from build123d import *

# Parameters (mm, degrees)
SKETCH2_W           = 18
SKETCH2_H           = 18
BOSS_EXTRUDE1_DEPTH = 8
BOSS_EXTRUDE1_TAPER = 11
FILLET1_R           = 1
SHELL1_OUTLINE_W    = 13.241242282
SHELL1_OUTLINE_H    = 13.241242282
SHELL1_DEPTH        = 7
SHELL1_DRAFT        = 11
SKETCH3_R           = 2.8
BOSS_EXTRUDE2_DEPTH = 5.5
SKETCH4_W           = 1.161559242
SKETCH4_H           = 1.419220379
SKETCH4_H_2         = 1.161559242
SKETCH4_W_2         = 1.419220379
CUT_EXTRUDE1_DEPTH  = 5.5


# Read off the part's stored shape, not the designer's step: Shell1
with BuildPart() as part:
    # Sketch2 → Boss-Extrude1 (new body)
    with BuildSketch(Plane(origin=(0, 0, 0), x_dir=(1, 0, 0), z_dir=(0, 1, 0))):
        Rectangle(SKETCH2_W, SKETCH2_H)
    extrude(amount=BOSS_EXTRUDE1_DEPTH, taper=BOSS_EXTRUDE1_TAPER)

    # Fillet1
    fillet1_edges = [part.edges().sort_by_distance(p)[0] for p in [
        (-7.444957527, 8, 0),
        (0, 8, 7.444957527),
        (7.444957527, 8, 0),
        (8.222478763, 4, 8.222478763),
        (-8.222478763, 4, 8.222478763),
        (-8.222478763, 4, -8.222478763),
        (8.222478763, 4, -8.222478763),
        (0, 8, -7.444957527),
    ]]
    fillet(fillet1_edges, radius=FILLET1_R)


with BuildPart() as shell1_tool:
    # Shell1 outline → Shell1 (with draft: the straight prism first)
    with BuildSketch(Plane(origin=(0, 7, 0), x_dir=(1, 0, 0), z_dir=(0, 1, 0))):
        Rectangle(SHELL1_OUTLINE_W, SHELL1_OUTLINE_H)
    extrude(amount=-SHELL1_DEPTH)
    # Shell1: the draft: its side faces are tilted about the plane it starts from
    shell1_sides = [shell1_tool.faces().sort_by_distance(p)[0] for p in [
        (0, 3.5, -6.620621141),
        (-6.620621141, 3.5, 0),
        (0, 3.5, 6.620621141),
        (6.620621141, 3.5, 0),
    ]]
    draft(shell1_sides, Plane(origin=(0, 7, 0), x_dir=(1, 0, 0), z_dir=(0, 1, 0)), SHELL1_DRAFT)


with BuildPart() as part_1:
    add(part.part)

    # Shell1: cut by shell1_tool
    add(shell1_tool.part, mode=Mode.SUBTRACT)

    # Sketch3 → Boss-Extrude2 (add)
    with BuildSketch(Plane.XZ.offset(-7)):
        with Locations(Location((0, 0, 0), (0, 0, 270))):
            Circle(SKETCH3_R)
    extrude(amount=BOSS_EXTRUDE2_DEPTH)

    # Sketch4 → Cut-Extrude1 (cut)
    with BuildSketch(Plane.XZ.offset(-1.5)):
        with Locations((0, -1.290389811)):
            Rectangle(SKETCH4_W, SKETCH4_H)
        Rectangle(SKETCH4_W, SKETCH4_H_2)
        with Locations((-1.290389811, 0)):
            Rectangle(SKETCH4_W_2, SKETCH4_H_2)
        with Locations((1.290389811, 0)):
            Rectangle(SKETCH4_W_2, SKETCH4_H_2)
        with Locations((0, 1.290389811)):
            Rectangle(SKETCH4_W, SKETCH4_H)
    extrude(amount=-CUT_EXTRUDE1_DEPTH, mode=Mode.SUBTRACT)


solid = part_1.part
Part model, mm, in its own coordinate system. A direction names the side the tool comes from. Give positions to 0.01 mm unless a question says otherwise; leave off trailing zeros. Use one line per item in the form item = value.
(1) Flat gauge pins, fed straight in: P1, Ø0.7, axis at y = 4.5, z = -1, coming from the -X side; P2, Ø1.3, axis at x = 0, y = 4.5, coming from the -Z side; P3, Ø1.6, axis at y = 3.5, z = 1.5, coming from the +X side. Where does each tip first touch, or does it go through?
Solution:
P1 = -8.19
P2 = -8.25
P3 = 8.48
(2) Pull direction X, two halves, no side cores. Call faces 3 (the face through (-0.581, 4, 1)), 4 (the face through (0, 8, 0)): +X half, -X half, draft (parallel to the pull), parting line (faces both ways), or undercut.
Solution:
face_3 = undercut
face_4 = draft
(3) Tool access for faces 1 (the face through (8.3, 0, 0.6)), 2 (the face through (-2, 4, 0)): list every direction of +Z, -Z, +X, -X, +Y, -Y with a clear straight run to the whole face (end or side of a thin tool).
Solution:
face_1 = +Z, -Z, +X, -X, -Y
face_2 = -Y
(4) Saw through at A-A (y = 4.5). Count the separate pieces of the cut face and the enclosed holes in it, then the cut area to 3 significant figures.
Solution:
separate_pieces = 2
enclosed_holes = 2
area = 77.9 mm²
(5) Drill centre lines: line 1 (X direction, y = 3.5, z = -1); line 2 (X direction, y = 3.5, z = -0.5) (3 decimals); line 3 (Z direction, x = -0.75, y = 3.5). Where is each one in solid material? Low to high. Write a range as from..to.
Solution:
line_1 = -8.32..-7.3, -2.62..-0.58, 0.58..2.62, 7.3..8.32
line_2 = -8.32..-7.301, -2.755..-2, 2..2.755, 7.301..8.32
line_3 = -8.32..-7.3, -2.7..-0.58, 0.58..2.7, 7.3..8.32
